from build123d import *

# Parameters (mm, degrees)
SKETCH1_W                = 46
SKETCH1_H                = 22
BOSS_EXTRUDE1_DEPTH      = 23
BOSS_EXTRUDE2_DEPTH      = 4.5
BOSS_EXTRUDE2_DEPTH_BACK = 26.5
SKETCH2_R                = 19
FILLET1_R                = 3


with BuildPart() as part:
    # Sketch1 → Boss-Extrude1 (new, symmetric)
    with BuildSketch(Plane(origin=(0, 0, 0), x_dir=(1, 0, 0), z_dir=(0, 1, 0))):
        Rectangle(SKETCH1_W, SKETCH1_H)
    extrude(amount=BOSS_EXTRUDE1_DEPTH, both=True)

    # Sketch2 → Boss-Extrude2 (add, two sides: drawn at the far end of the back side and taken through both)
    with BuildSketch(Plane.XY.offset(11).offset(-BOSS_EXTRUDE2_DEPTH_BACK)):
        Circle(SKETCH2_R)
    extrude(amount=BOSS_EXTRUDE2_DEPTH + BOSS_EXTRUDE2_DEPTH_BACK)

    # Sketch3 → Cut-Revolve1 (revolve, cut)
    with BuildSketch(Plane(origin=(0, 0, 0), x_dir=(1, 0, 0), z_dir=(0, 1, 0)), mode=Mode.PRIVATE) as cut_revolve1_sk:
        Polygon((0, 15.5), (0, -15.5), (12.5, -15.5), (12.5, 12.5), (16, 12.5), (16, 15.5), align=None)
    revolve(cut_revolve1_sk.sketch.rotate(Axis((0, 0, -15.5), (0, 0, 1)), 180), axis=Axis((0, 0, -15.5), (0, 0, 1)), mode=Mode.SUBTRACT)

    # Sketch4 → Revolve1 (revolve)
    with BuildSketch(Plane(origin=(0, 0, 0), x_dir=(1, 0, 0), z_dir=(0, 1, 0))):
        Polygon((-45, 0), (-45, 6), (-35, 6), (-35, 8), (-23, 8), (-23, 0), align=None)
    revolve1 = revolve(axis=Axis((-23, 0, 0), (-1, 0, 0)))

    # Mirror1: Revolve1 across plane
    add(revolve1.mirror(Plane(origin=(0, 0, 0), x_dir=(0, 0, 1), z_dir=(1, 0, 0))))

    # Fillet1
    fillet1_edges = [part.edges().sort_by_distance(p)[0] for p in [
        (-19, 0, -11),
        (-19, 0, 11),
    ]]
    fillet(fillet1_edges, radius=FILLET1_R)


solid = part.part
Read the model definition and answer for the solid it produces. Units are mm, in the model's axes. A direction names the side the tool comes from. Round coordinates to 2 decimals unless told otherwise and drop trailing zeros. Order: outer loops, then holes, each group sorted by start corner. A loop starts at its lowest first (then second) coordinate and runs counter-clockwise, first axis right, second up.
1) For faces 4 (the face through (35, -6, -2)), 5 (the face through (-12, -19, 11)), 6 (the face through (-40, 0, 6)), 7 (the face through (-12, -19, -11)), determine the directions among +Z, -Z, +X, -X, +Y, -Y from which every point of the face is accessible in a straight line to the end or side of a thin tool.
2) The part is cut by section B-B on x = 0. Write down the section's boundary in (y, z), plus the area to 3 significant figures.
3) Flat-ended cylindrical pins translate along their axes: pin 1 (8 mm diameter, centred on y = 10.5, z = 6, fed in from -X); pin 2 (1.5 mm diameter, centred on y = 15.5, z = 6.5, fed in from +X). Find the tip coordinate at first contact, or state that the pin passes through.
4) The part is cut by section C-C on x = -33.5. Write down the section's boundary in (y, z), plus the area to 3 significant figures.
5) The mould has two halves that part along Y. Classify faces 1 (the face through (23, 5, 7)), 2 (the face through (28.92, 7.81, 1.73)), 3 (the face through (-11.923, -3.755, 1.304)): released by +Y, released by -Y, zero draft, split by the parting line, or undercut.
6) The part is cut by section A-A on z = 0. Write down the section's boundary in (x, y), plus the area to 3 significant figures.
7) Straight lines are drawn through the part: L1, parallel to Y at x = 0, z = 9; L2, parallel to Y at x = 0, z = -14.9; L3, parallel to X at y = -20, z = -0.5. For each, find the intervals that lie inside material, in ascending order.
8) The part is cut by section D-D on x = 39.5. Write down the section's boundary in (y, z).
Resolved:
1. face 4: +X
1. face 5: +Z
1. face 6: -X
1. face 7: -Z
2. outline: (-23, -11) - (-22, -11) arc R3 cw to (-19, -14) - (-19, -15.5) - (-16, -15.5) - (-16, -12.5) - (-12.5, -12.5) - (-12.5, 15.5) - (-19, 15.5) - (-19, 14) arc R3 cw to (-22, 11) - (-23, 11) - close; (12.5, -12.5) - (16, -12.5) - (16, -15.5) - (19, -15.5) - (19, -14) arc R3 cw to (22, -11) - (23, -11) - (23, 11) - (22, 11) arc R3 cw to (19, 14) - (19, 15.5) - (12.5, 15.5) - close
2. area: 566 mm2
3. pin 1: stops at x = -23
3. pin 2: stops at x = 23
4. outline: circle Ø16 at (0, 0)
4. area: 201 mm2
5. face 1: zero draft
5. face 2: split by the parting line
5. face 3: undercut
6. outline: (-45, -6) - (-35, -6) - (-35, -8) - (-23, -8) - (-23, -23) - (23, -23) - (23, -8) - (35, -8) - (35, -6) - (45, -6) - (45, 6) - (35, 6) - (35, 8) - (23, 8) - (23, 23) - (-23, 23) - (-23, 8) - (-35, 8) - (-35, 6) - (-45, 6) - close; hole circle Ø25 at (0, 0)
6. area: 2,250 mm2
7. L1: y = -23 to -12.5, 12.5 to 23
7. L2: y = -19 to -16, 16 to 19
7. L3: x = -23 to 23
8. outline: circle Ø12 at (0, 0)
